Work out the finished part from the listing and answer in its coordinate system (mm). Face numbers are marked on the shaded views. A direction names the side the tool comes from. Give positions to 0.01 mm unless a question says otherwise; leave off trailing zeros. Write each loop counter-clockwise with the first axis right and the second up, starting at its lowest first coordinate (ties: lowest second). Pieces come first, ordered by that corner, then holes. Notation, with made-up numbers: (10, -5.5) -> (33, -5.5) arc R16 cw to (33, 19.5) -> close; hole circle Ø8 at (52, 60.5). An arc over 180 degrees is marked (long way). Use a Markdown table: item, result. Add a question column.
Q1. Section A-A, the plane z = 42.5 is taken. Give the vertices of the cut face in (x, y), plus the area to 3 significant figures.
Q2. Each of these flat-tipped pins is pushed along its axis until it touches: pin 1 Ø7 at (x, y) = (1, 8.5) entering from +Z; pin 2 Ø14.5 at (y, z) = (27.5, -19.5) entering from +X; pin 3 Ø5 at (x, z) = (0.5, 62) entering from +Y; pin 4 Ø4.5 at (x, z) = (7, -45.5) entering from +Y. Where does it stop, or does it pass through?
Q3. For the marked faces 1, 2, 3, 4 and 5, determine the directions among +Z, -Z, +X, -X, +Y, -Y from which every point of the face is accessible in a straight line to the end or side of a thin tool.
Q4. Consider line 1 (X direction, y = 13, z = 26); line 2 (X direction, y = 28, z = 57); line 3 (X direction, y = 24.5, z = -26). Determine where each line is inside the solid, lowest interval first.
Q5. For a pull along Z with two mould halves and no side action, classify the marked faces 6, 7, 8 and 9 as pulls with the +Z half, pulls with the -Z half, needs draft (parallel to the pull), parting line crosses it, or undercut.
Q6. Section C-C, the plane z = 64.5 is taken. Give the vertices of the cut face in (x, y), plus the area to 3 significant figures.
Q7. Section B-B, the plane y = 7.5 is taken. Give the vertices of the cut face in (x, z), plus the area to 3 significant figures.
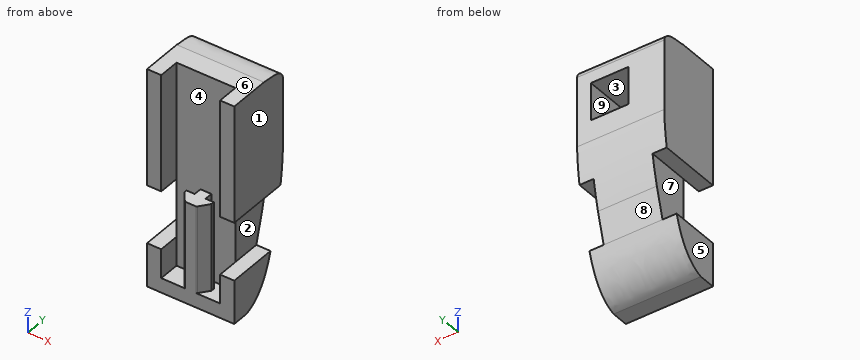
from build123d import *

# Parameters (mm, degrees)
SKETCH_1_W                = 100
SKETCH_1_H                = 185
EXTRUDE_1_DEPTH           = 100
SKETCH_2_W                = 100
SKETCH_2_H                = 3.8
CUT_EXTRUDE_1_DEPTH       = 155
CUT_EXTRUDE_2_DEPTH       = 155
SKETCH_4_W                = 25.5
SKETCH_4_H                = 25.5
CUT_EXTRUDE_3_DEPTH       = 79
SKETCH_6_W                = 89.706259743
SKETCH_6_H                = 10
SKETCH_6_W_2              = 10.293740257
CUT_EXTRUDE_4_DEPTH       = 146.107718609
CUT_EXTRUDE_5_DEPTH       = 169.985946161
CUT_EXTRUDE_5_DEPTH_BACK  = 169.985946161
SKETCH_7_W                = 20
SKETCH_7_H                = 3.8
EXTRUDE_4_DEPTH           = 160
SKETCH_10_W               = 16
SKETCH_10_H               = 1.8
CUT_EXTRUDE_6_DEPTH       = 155
SKETCH_13_W               = 20
SKETCH_13_H               = 175
CUT_EXTRUDE_7_DEPTH       = 143.515578096
SKETCH_14_W               = 175
SKETCH_14_H               = 50
CUT_EXTRUDE_8_DEPTH       = 149.849756466
SKETCH_15_W               = 60
SKETCH_15_H               = 10
CUT_EXTRUDE_9_DEPTH       = 108.660066877
SKETCH_16_W               = 60
SKETCH_16_H               = 14.5
CUT_EXTRUDE_10_DEPTH      = 108.660066877
CUT_EXTRUDE_11_DEPTH      = 111.381157812
CUT_EXTRUDE_21_DEPTH      = 162.400898529
CUT_EXTRUDE_21_DEPTH_BACK = 140.5
CUT_EXTRUDE_26_DEPTH      = 111.381157983
SKETCH_34_W               = 10
SKETCH_34_H               = 20
CUT_EXTRUDE_31_DEPTH      = 96.490523251
SKETCH_35_W               = 18.74373947
SKETCH_35_H               = 80.5
CUT_EXTRUDE_32_DEPTH      = 14
CUT_EXTRUDE_35_DEPTH      = 60
CUT_EXTRUDE_36_DEPTH      = 140.5
SKETCH_43_W               = 0.25
SKETCH_43_H               = 0.002112168
CUT_EXTRUDE_37_DEPTH      = 140.5
SKETCH_44_W               = 7.5
SKETCH_44_H               = 0.502112168
CUT_EXTRUDE_38_DEPTH      = 80.4999
SKETCH_45_W               = 9.75
SKETCH_45_H               = 20
SKETCH_45_W_2             = 9.75146362
CUT_EXTRUDE_39_DEPTH      = 96.490523251
SKETCH_46_W               = 0.24853638
SKETCH_46_H               = 20
SKETCH_46_W_2             = 0.25
EXTRUDE_5_DEPTH           = 31.697888
CUT_EXTRUDE_40_DEPTH      = 106.399537724
CUT_EXTRUDE_40_DEPTH_BACK = 106.399537724
SKETCH_54_W               = 25.5
SKETCH_54_H               = 0.5
CUT_EXTRUDE_41_DEPTH      = 29
SKETCH_55_W               = 26
SKETCH_55_H               = 26
EXTRUDE_6_DEPTH           = 29
SKETCH_56_W               = 25.8
SKETCH_56_H               = 25.8
CUT_EXTRUDE_42_DEPTH      = 29


with BuildPart() as part:
    # 草图1 → 凸台-拉伸1 (new body)
    with BuildSketch(Plane(origin=(0, 0, 0), x_dir=(1, 0, 0), z_dir=(0, 1, 0))):
        Rectangle(SKETCH_1_W, SKETCH_1_H)
    extrude(amount=EXTRUDE_1_DEPTH)

    # 草图2 → 切除-拉伸1 (cut)
    with BuildSketch(Plane.XY.offset(92.5)):
        with Locations((0, 1.9)):
            Rectangle(SKETCH_2_W, SKETCH_2_H)
    extrude(amount=-CUT_EXTRUDE_1_DEPTH, mode=Mode.SUBTRACT)

    # 草图3 → 切除-拉伸2 (cut)
    with BuildSketch(Plane.XY.offset(92.5)):
        with BuildLine():
            Line((-20, 3.8), (-3.51, 3.8))
            ThreePointArc((-3.51, 3.8), (-3.949598778, 3.901619975), (-4.3, 4.185860522))
            Line((-4.3, 4.185860522), (-9.371869735, 10.69267521))
            ThreePointArc((-9.371869735, 10.69267521), (-9.267749528, 11.143089764), (-8.9765156, 11.502112168))
            Line((-8.9765156, 11.502112168), (-4.5, 11.502112168))
            ThreePointArc((-4.5, 11.502112168), (-4.146446609, 11.648558777), (-4, 12.002112168))
            Line((-4, 12.002112168), (-4, 16.002112168))
            Line((-4, 16.002112168), (-20, 16.002112168))
            Line((-20, 16.002112168), (-20, 3.8))
        make_face()
        with BuildLine():
            ThreePointArc((4.3, 4.185860522), (3.949598778, 3.901619975), (3.51, 3.8))
            Line((3.51, 3.8), (20, 3.8))
            Line((20, 3.8), (20, 16.002112168))
            Line((20, 16.002112168), (4, 16.002112168))
            Line((4, 16.002112168), (4, 12.002112168))
            ThreePointArc((4, 12.002112168), (4.146446609, 11.648558777), (4.5, 11.502112168))
            Line((4.5, 11.502112168), (8.9765156, 11.502112168))
            ThreePointArc((8.9765156, 11.502112168), (9.426930154, 11.220838522), (9.371869735, 10.69267521))
            Line((9.371869735, 10.69267521), (4.3, 4.185860522))
        make_face()
    extrude(amount=-CUT_EXTRUDE_2_DEPTH, mode=Mode.SUBTRACT)

    # 草图4 → 切除-拉伸3 (cut)
    with BuildSketch(Plane(origin=(0, 100, 0), x_dir=(1, 0, 0), z_dir=(0, 1, 0))):
        with Locations((7.75, -50.25)):
            Rectangle(SKETCH_4_W, SKETCH_4_H)
    extrude(amount=-CUT_EXTRUDE_3_DEPTH, mode=Mode.SUBTRACT)

    # 草图6 → 切除-拉伸4 (cut, through all)
    with BuildSketch(Plane(origin=(0, 100, 0), x_dir=(1, 0, 0), z_dir=(0, 1, 0))):
        with Locations((5.146870128, 87.5)):
            Rectangle(SKETCH_6_W, SKETCH_6_H)
        with Locations((-44.853129872, 87.5)):
            Rectangle(SKETCH_6_W_2, SKETCH_6_H)
    extrude(amount=-CUT_EXTRUDE_4_DEPTH, mode=Mode.SUBTRACT)

    # 草图7 → 切除-拉伸5 (cut, two sides: drawn at the far end of the back side and taken through both)
    with BuildSketch(Plane.ZY.offset(50).offset(-CUT_EXTRUDE_5_DEPTH_BACK)):
        with Locations((-72.5, 1.9)):
            Rectangle(SKETCH_7_W, SKETCH_7_H)
    extrude(amount=CUT_EXTRUDE_5_DEPTH + CUT_EXTRUDE_5_DEPTH_BACK, mode=Mode.SUBTRACT)

    # 草图9 → 凸台-拉伸4 (add)
    with BuildSketch(Plane.XY.offset(92.5)):
        Polygon((-9.371869735, 10.69267521), (-9.371869735, 13.29267521), (-4, 13.29267521), (4, 13.29267521), (9.371869735, 13.29267521), (9.371869735, 10.69267521), align=None)
    extrude(amount=-EXTRUDE_4_DEPTH)

    # 草图10 → 切除-拉伸6 (cut)
    with BuildSketch(Plane.XY.offset(92.5)):
        with Locations((-12, 16.902112168)):
            Rectangle(SKETCH_10_W, SKETCH_10_H)
        Polygon((4, 16.002112168), (4, 17.802112168), (19.99853638, 17.802112168), (20, 16.002112168), align=None)
    extrude(amount=-CUT_EXTRUDE_6_DEPTH, mode=Mode.SUBTRACT)

    # 草图13 → 切除-拉伸7 (cut, through all)
    with BuildSketch(Plane.XZ.offset(-3.8)):
        with Locations((-40, 5)):
            Rectangle(SKETCH_13_W, SKETCH_13_H)
        with Locations((40, 5)):
            Rectangle(SKETCH_13_W, SKETCH_13_H)
    extrude(amount=-CUT_EXTRUDE_7_DEPTH, mode=Mode.SUBTRACT)

    # 草图14 → 切除-拉伸8 (cut, through all)
    with BuildSketch(Plane(origin=(30, 0, 0), x_dir=(0, 0, -1), z_dir=(1, 0, 0))):
        with Locations((-5, 75)):
            Rectangle(SKETCH_14_W, SKETCH_14_H)
    extrude(amount=-CUT_EXTRUDE_8_DEPTH, mode=Mode.SUBTRACT)

    # 草图15 → 切除-拉伸9 (cut, through all)
    with BuildSketch(Plane.XZ.offset(-3.8)):
        with Locations((0, -77.5)):
            Rectangle(SKETCH_15_W, SKETCH_15_H)
    extrude(amount=-CUT_EXTRUDE_9_DEPTH, mode=Mode.SUBTRACT)

    # 草图16 → 切除-拉伸10 (cut, through all)
    with BuildSketch(Plane(origin=(0, 50, 0), x_dir=(1, 0, 0), z_dir=(0, 1, 0))):
        with Locations((0, -85.25)):
            Rectangle(SKETCH_16_W, SKETCH_16_H)
    extrude(amount=-CUT_EXTRUDE_10_DEPTH, mode=Mode.SUBTRACT)

    # 草图17 → 切除-拉伸11 (cut, through all)
    with BuildSketch(Plane(origin=(30, 0, 0), x_dir=(0, 0, -1), z_dir=(1, 0, 0))):
        with BuildLine():
            Line((72.5, 50), (-22.5, 50))
            add(Edge.make_bspline(
                [(-22.5, 50), (-9.330669895, 49.706144403), (11.085821801, 46.827148239), (38.239751221, 39.498978447), (59.688603115, 33.272875951), (70.679662454, 22.295526596), (72.5, 15.311284203)],
                knots=[0, 0, 0, 0, 0.374533404, 0.581855131, 0.802431491, 1, 1, 1, 1], degree=3))
            Line((72.5, 15.311284203), (72.5, 50))
        make_face()
    extrude(amount=-CUT_EXTRUDE_11_DEPTH, mode=Mode.SUBTRACT)

    # 草图24 → 切除-拉伸21 (cut, two sides: drawn at the far end of the back side and taken through both)
    with BuildSketch(Plane.XY.offset(78).offset(-CUT_EXTRUDE_21_DEPTH_BACK)):
        with BuildLine():
            Line((9.371869735, 11.309008937), (9.371869735, 10.69267521))
            ThreePointArc((9.371869735, 10.69267521), (9.477785695, 11.000842073), (9.371869735, 11.309008937))
        make_face()
    extrude(amount=CUT_EXTRUDE_21_DEPTH + CUT_EXTRUDE_21_DEPTH_BACK, mode=Mode.SUBTRACT)

    # 草图28 → 切除-拉伸26 (cut, through all)
    with BuildSketch(Plane(origin=(30, 0, 0), x_dir=(0, 0, -1), z_dir=(1, 0, 0))):
        with BuildLine():
            Line((-70.5, 50), (-78, 50))
            Line((-78, 50), (-78, 31.982866201))
            add(Edge.make_bspline(
                [(-70.5, 50), (-78.410932033, 48.656434308), (-77.0737544, 36.843285786), (-78, 31.982866201)],
                knots=[0, 0, 0, 0, 1, 1, 1, 1], degree=3))
        make_face()
    extrude(amount=-CUT_EXTRUDE_26_DEPTH, mode=Mode.SUBTRACT)

    # 草图34 → 切除-拉伸31 (cut, through all)
    with BuildSketch(Plane.XZ.offset(-3.8)):
        with Locations((-25, -32.5)):
            Rectangle(SKETCH_34_W, SKETCH_34_H)
        with Locations((25, -32.5)):
            Rectangle(SKETCH_34_W, SKETCH_34_H)
    extrude(amount=-CUT_EXTRUDE_31_DEPTH, mode=Mode.SUBTRACT)

    # 草图35 → 切除-拉伸32 (cut)
    with BuildSketch(Plane.XZ.offset(-3.8)):
        with Locations((0, 37.75)):
            Rectangle(SKETCH_35_W, SKETCH_35_H)
    extrude(amount=-CUT_EXTRUDE_32_DEPTH, mode=Mode.SUBTRACT)

    # 草图40 → 切除-拉伸35 (cut)
    with BuildSketch(Plane.XY.offset(-2.5)):
        Polygon((4, 13.29267521), (4, 17.8), (3.75, 17.8), (3.75, 12.79267521), (9.371869735, 12.79267521), (9.371869735, 13.29267521), align=None)
        Polygon((-3.75, 17.8), (-4, 17.8), (-4, 13.29267521), (-9.371869735, 13.29267521), (-9.371869735, 12.79267521), (-3.75, 12.79267521), align=None)
    extrude(amount=-CUT_EXTRUDE_35_DEPTH, mode=Mode.SUBTRACT)

    # 草图41 → 切除-拉伸36 (cut)
    with BuildSketch(Plane.XY.offset(78)):
        Polygon((-3.75, 18.302112168), (-20.25, 18.302112168), (-20.25, 3.8), (-20, 3.8), (-20, 17.802112168), (-3.75, 17.802112168), align=None)
        Polygon((3.75, 18.302112168), (3.75, 17.802112168), (19.99853638, 17.802112168), (19.99853638, 3.8), (20.24853638, 3.8), (20.24853638, 18.302112168), align=None)
    extrude(amount=-CUT_EXTRUDE_36_DEPTH, mode=Mode.SUBTRACT)

    # 草图43 → 切除-拉伸37 (cut)
    with BuildSketch(Plane.XY.offset(78)):
        with Locations((-3.875, 17.801056084)):
            Rectangle(SKETCH_43_W, SKETCH_43_H)
        with Locations((3.875, 17.801056084)):
            Rectangle(SKETCH_43_W, SKETCH_43_H)
    extrude(amount=-CUT_EXTRUDE_37_DEPTH, mode=Mode.SUBTRACT)

    # 草图44 → 切除-拉伸38 (cut)
    with BuildSketch(Plane.XY.offset(78)):
        with Locations((0, 18.051056084)):
            Rectangle(SKETCH_44_W, SKETCH_44_H)
    extrude(amount=-CUT_EXTRUDE_38_DEPTH, mode=Mode.SUBTRACT)

    # 草图45 → 切除-拉伸39 (cut, through all)
    with BuildSketch(Plane.XZ.offset(-3.8)):
        with Locations((-25.125, -12.5)):
            Rectangle(SKETCH_45_W, SKETCH_45_H)
        with Locations((25.12426819, -12.5)):
            Rectangle(SKETCH_45_W_2, SKETCH_45_H)
    extrude(amount=-CUT_EXTRUDE_39_DEPTH, mode=Mode.SUBTRACT)

    # 草图46 → 凸台-拉伸5 (add, through all)
    with BuildSketch(Plane.XZ.offset(-18.302112168)):
        with Locations((20.12426819, -32.5)):
            Rectangle(SKETCH_46_W, SKETCH_46_H)
        with Locations((-20.125, -32.5)):
            Rectangle(SKETCH_46_W_2, SKETCH_46_H)
    extrude(amount=-EXTRUDE_5_DEPTH)

    # 草图47 → 切除-拉伸40 (cut, two sides: drawn at the far end of the back side and taken through both)
    with BuildSketch(Plane.ZY.offset(20.25).offset(-CUT_EXTRUDE_40_DEPTH_BACK)):
        Polygon((-42.5, 38.203961841), (-22.5, 43.618048783), (-22.5, 50), (-42.5, 50), align=None)
    extrude(amount=CUT_EXTRUDE_40_DEPTH + CUT_EXTRUDE_40_DEPTH_BACK, mode=Mode.SUBTRACT)

    # 草图54 → 切除-拉伸41 (cut)
    with BuildSketch(Plane(origin=(0, 50, 0), x_dir=(1, 0, 0), z_dir=(0, 1, 0))):
        with Locations((7.75, -37.25)):
            Rectangle(SKETCH_54_W, SKETCH_54_H)
        Polygon((-5, -63), (-5, -37.5), (-5, -37), (-5.5, -37), (-5.5, -63), align=None)
    extrude(amount=-CUT_EXTRUDE_41_DEPTH, mode=Mode.SUBTRACT)

    # 草图55 → 凸台-拉伸6 (add)
    with BuildSketch(Plane(origin=(0, 50, 0), x_dir=(1, 0, 0), z_dir=(0, 1, 0))):
        with Locations((7.5, -50)):
            Rectangle(SKETCH_55_W, SKETCH_55_H)
    extrude(amount=-EXTRUDE_6_DEPTH)

    # 草图56 → 切除-拉伸42 (cut)
    with BuildSketch(Plane(origin=(0, 50, 0), x_dir=(1, 0, 0), z_dir=(0, 1, 0))):
        with Locations((7.6, -49.7)):
            Rectangle(SKETCH_56_W, SKETCH_56_H)
    extrude(amount=-CUT_EXTRUDE_42_DEPTH, mode=Mode.SUBTRACT)


solid = part.part
Result set:
| question | item | result |
|---|---|---|
| 1 | outline | (-30, 3.8) -> (-20.25, 3.8) -> (-20.25, 18.3) -> (20.25, 18.3) -> (20.25, 3.8) -> (30, 3.8) -> (30, 50) -> (20.5, 50) -> (20.5, 21) -> (-5.3, 21) -> (-5.3, 50) -> (-30, 50) -> close |
| 1 | area | 1,440 mm2 |
| 2 | pin 1 | stops at z = -2.5 |
| 2 | pin 2 | stops at x = 20.25 |
| 2 | pin 3 | stops at y = 50 |
| 2 | pin 4 | stops at y = 37.98 |
| 3 | face 1 | +Z, -Z, +X, +Y, -Y |
| 3 | face 2 | +X, +Y, -Y |
| 3 | face 3 | +Y |
| 3 | face 4 | +Z |
| 3 | face 5 | +Z, -Z, -X, +Y, -Y |
| 4 | line 1 | x = -30 to -20.25, 20.25 to 30 |
| 4 | line 2 | x = -30 to -5.3, 20.5 to 30 |
| 4 | line 3 | x = -20.25 to 20.25 |
| 5 | face 6 | pulls with the +Z half |
| 5 | face 7 | undercut |
| 5 | face 8 | pulls with the -Z half |
| 5 | face 9 | undercut |
| 6 | outline | (-30, 3.8) -> (-20.25, 3.8) -> (-20.25, 18.3) -> (20.25, 18.3) -> (20.25, 3.8) -> (30, 3.8) -> (30, 50) -> (-30, 50) -> close |
| 6 | area | 2,180 mm2 |
| 7 | outline | (-30, -72.5) -> (30, -72.5) -> (30, -42.5) -> (20.25, -42.5) -> (20.25, -62.5) -> (6.88, -62.5) -> (6.88, -2.5) -> (-6.88, -2.5) -> (-6.88, -62.5) -> (-20.25, -62.5) -> (-20.25, -42.5) -> (-30, -42.5) -> close; (-30, -2.5) -> (-20.25, -2.5) -> (-20.25, 78) -> (-30, 78) -> close; (20.25, -2.5) -> (30, -2.5) -> (30, 78) -> (20.25, 78) -> close |
| 7 | area | 3,390 mm2 |
